from build123d import *

# Parameters (mm, degrees)
F0_W     = 203.2
F0_H     = 63.5
F1_DEPTH = 25.4
F2_R     = 9.525
F3_DEPTH = 12.7
F4_W     = 190.5
F4_H     = 50.8
F5_DEPTH = 3.175


with BuildPart() as f1:
    # F0 (on Top) → F1 (new body)
    with BuildSketch(Plane.XY):
        Rectangle(F0_W, F0_H)
    extrude(amount=F1_DEPTH)

    # F2 (on face) → F3 (cut)
    with BuildSketch(Plane(origin=(0, 0, 0), x_dir=(1, 0, 0), z_dir=(0, 0, -1))):
        with Locations((-81.4832, 0)):
            Circle(F2_R)
        with Locations((71.3232, 0)):
            Circle(F2_R)
    extrude(amount=-F3_DEPTH, mode=Mode.SUBTRACT)

    # F4 (on face) → F5 (join)
    with BuildSketch(Plane.XY.offset(25.4)):
        Rectangle(F4_W, F4_H)
    extrude(amount=F5_DEPTH)


solid = f1.part
For this review, take the finished solid that the model builds, in its own axes (mm). A direction names the side the tool comes from. Give positions to 0.01 mm unless a question says otherwise; leave off trailing zeros. Order: outer loops, then holes, each group sorted by start corner. A loop starts at its lowest first (then second) coordinate and runs counter-clockwise, first axis right, second up. Notation, with made-up numbers: (55, 49) -> (107, 49) arc R22 cw to (107, 83) -> close; hole circle Ø10 at (-22, 85). An arc over 180 degrees is marked (long way). Write item = value, one per line.
1) For faces 5 (the face through (-101.6, 0, 13)), 6 (the face through (-82, 0, 12.7)), list the 3-axis set-ups (+Z, -Z, +X, -X, +Y, -Y) from which the entire face can be reached by the end or side of a thin tool; tool diameter is ignored.
Findings:
face_5 = +Z, -Z, -X, +Y, -Y
face_6 = -Z
2) Insertion check: pin 1 (17 mm diameter, centred on x = 71.32, y = 0, fed in from -Z); pin 2 (2.5 mm diameter, centred on y = -8, z = 27, fed in from -X); pin 3 (1.6 mm diameter, centred on x = 47, z = 27.5, fed in from +Y). Each pin has a flat end and moves straight along its axis. Give the tip position at first contact, or say it passes through.
Findings:
pin_1 = 12.7
pin_2 = -95.25
pin_3 = 25.4
3) Draft analysis for pull direction Y (two halves, no side actions). For faces 1 (the face through (71, 0, 12.7)), 2 (the face through (80.41, -2.86, 6.26)), 3 (the face through (101.6, 0, 13)), 4 (the face through (-1, 31.75, 13)), state which applies: pulls with the +Y half, pulls with the -Y half, needs draft (parallel to the pull), parting line crosses it, or undercut.
Findings:
face_1 = undercut
face_2 = undercut
face_3 = needs draft
face_4 = pulls with the +Y half
4) We need section B-B, the plane z = 3.25. Give the boundary of the cut face in (x, y) (3 decimals).
Findings:
outline = (-101.6, -31.75) -> (101.6, -31.75) -> (101.6, 31.75) -> (-101.6, 31.75) -> close; hole circle Ø19.05 at (-81.483, 0); hole circle Ø19.05 at (71.323, 0)
5) To check wall thickness, follow L1, parallel to X at y = 0, z = 8.25; L2, parallel to Z at x = -81.5, y = -27.5; L3, parallel to Z at x = 67, y = -3.5 (3 decimals). State the ranges of each line that lie inside material, in increasing order. Write a range as from..to.
Findings:
L1 = -101.6..-91.01, -71.96..61.8, 80.85..101.6
L2 = 0..25.4
L3 = 12.7..28.575
6) We need section A-A, the plane x = -42.5. Give the boundary of the cut face in (y, z) (3 decimals), and give its area (3 significant figures).
Findings:
outline = (-31.75, 0) -> (31.75, 0) -> (31.75, 25.4) -> (25.4, 25.4) -> (25.4, 28.575) -> (-25.4, 28.575) -> (-25.4, 25.4) -> (-31.75, 25.4) -> close
area = 1,770 mm^2
7) We need section C-C, the plane y = 0. Give the boundary of the cut face in (x, z) (3 decimals), and give its area (3 significant figures).
Findings:
outline = (-101.6, 0) -> (-91.008, 0) -> (-91.008, 12.7) -> (-71.958, 12.7) -> (-71.958, 0) -> (61.798, 0) -> (61.798, 12.7) -> (80.848, 12.7) -> (80.848, 0) -> (101.6, 0) -> (101.6, 25.4) -> (95.25, 25.4) -> (95.25, 28.575) -> (-95.25, 28.575) -> (-95.25, 25.4) -> (-101.6, 25.4) -> close
area = 5,280 mm^2
8) We need section D-D, the plane x = 78. Give the boundary of the cut face in (y, z) (3 decimals).
Findings:
outline = (-31.75, 0) -> (-6.793, 0) -> (-6.793, 12.7) -> (6.793, 12.7) -> (6.793, 0) -> (31.75, 0) -> (31.75, 25.4) -> (25.4, 25.4) -> (25.4, 28.575) -> (-25.4, 28.575) -> (-25.4, 25.4) -> (-31.75, 25.4) -> close
